Can you work these out from the model? Positions are in its coordinate system, mm. Face numbers are marked on the shaded views. Round coordinates to 2 decimals unless told otherwise and drop trailing zeros. Order: outer loops, then holes, each group sorted by start corner. A loop starts at its lowest first (then second) coordinate and runs counter-clockwise, first axis right, second up. Notation, with made-up numbers: (-14, 88.5) -> (23, 88.5) arc R14 cw to (23, 102.5) -> close; hole circle Ø9 at (26, -16.75). An arc over 180 degrees is marked (long way). Use a Markdown table: item, result. Add a question column.
Q1. I need wall thicknesses on line 1 along Y through (x, z) = (0, 3.4); line 2 along Y through (x, z) = (-14, 2.1); line 3 along X through (y, z) = (-18, 4.5). Which ranges of each line are inside material? Lowest first, please. Write a range as [from, to].
Q2. I'm going to push flat-ended pins straight in: pin 1 Ø2 at (x, y) = (0, 19) entering from -Z; pin 2 Ø2 at (y, z) = (-10, 2.5) entering from -X; pin 3 Ø2 at (y, z) = (7, 3) entering from +X. Where does each tip first touch, or does it pass through?
Q3. If we section it at D-D on z = 2.25: Give the number of separate pieces and of enclosed holes in the cut face, plus the area to 3 significant figures.
Q4. If we section it at B-B on y = 0: List the corners of the cut face in (x, z) for me.
Q5. If we section it at A-A on x = 0: List the corners of the cut face in (y, z) for me.
Q6. If we section it at C-C on x = 5: List the corners of the cut face in (y, z) for me, plus the area to 3 significant figures.
Q7. We'd pull the mould along X, two halves only. Please class the marked faces 1, 2 and 3: +X half, -X half, draft (parallel to the pull), parting line (faces both ways), or undercut.
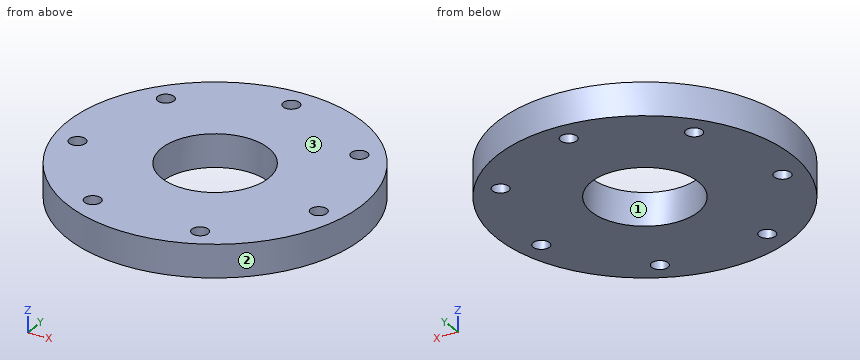
```python
from build123d import *

# Parameters (mm, degrees)
SKETCH1_R           = 22.5
SKETCH1_R_2         = 1.25
SKETCH1_R_3         = 8.15
BOSS_EXTRUDE1_DEPTH = 5


with BuildPart() as part:
    # Sketch1 → Boss-Extrude1 (new body)
    with BuildSketch(Plane.XY):
        Circle(SKETCH1_R)
        with Locations((0, 19)):
            Circle(SKETCH1_R_2, mode=Mode.SUBTRACT)
        with Locations((14.854798167, 11.846306235)):
            Circle(SKETCH1_R_2, mode=Mode.SUBTRACT)
        with Locations((18.523630331, -4.227897745)):
            Circle(SKETCH1_R_2, mode=Mode.SUBTRACT)
        with Locations((8.243791043, -17.11840849)):
            Circle(SKETCH1_R_2, mode=Mode.SUBTRACT)
        with Locations((-8.243791043, -17.11840849)):
            Circle(SKETCH1_R_2, mode=Mode.SUBTRACT)
        with Locations((-18.523630331, -4.227897745)):
            Circle(SKETCH1_R_2, mode=Mode.SUBTRACT)
        Circle(SKETCH1_R_3, mode=Mode.SUBTRACT)
        with Locations((-14.854798167, 11.846306235)):
            Circle(SKETCH1_R_2, mode=Mode.SUBTRACT)
    extrude(amount=BOSS_EXTRUDE1_DEPTH)


solid = part.part
```
Answer below:
| question | item | result |
|---|---|---|
| 1 | line 1 | [-22.5, -8.15], [8.15, 17.75], [20.25, 22.5] |
| 1 | line 2 | [-17.61, 10.93], [12.76, 17.61] |
| 1 | line 3 | [-13.5, -9.13], [-7.36, 7.36], [9.13, 13.5] |
| 2 | pin 1 | through |
| 2 | pin 2 | x = -20.62 |
| 2 | pin 3 | x = 21.69 |
| 3 | separate pieces | 1 |
| 3 | enclosed holes | 8 |
| 3 | area | 1,350 mm² |
| 4 | outline | (-22.5, 0) -> (-8.15, 0) -> (-8.15, 5) -> (-22.5, 5) -> close; (8.15, 0) -> (22.5, 0) -> (22.5, 5) -> (8.15, 5) -> close |
| 5 | outline | (-22.5, 0) -> (-8.15, 0) -> (-8.15, 5) -> (-22.5, 5) -> close; (8.15, 0) -> (17.75, 0) -> (17.75, 5) -> (8.15, 5) -> close; (20.25, 0) -> (22.5, 0) -> (22.5, 5) -> (20.25, 5) -> close |
| 6 | outline | (-21.94, 0) -> (-6.44, 0) -> (-6.44, 5) -> (-21.94, 5) -> close; (6.44, 0) -> (21.94, 0) -> (21.94, 5) -> (6.44, 5) -> close |
| 6 | area | 155 mm² |
| 7 | face 1 | undercut |
| 7 | face 2 | parting line |
| 7 | face 3 | draft |
